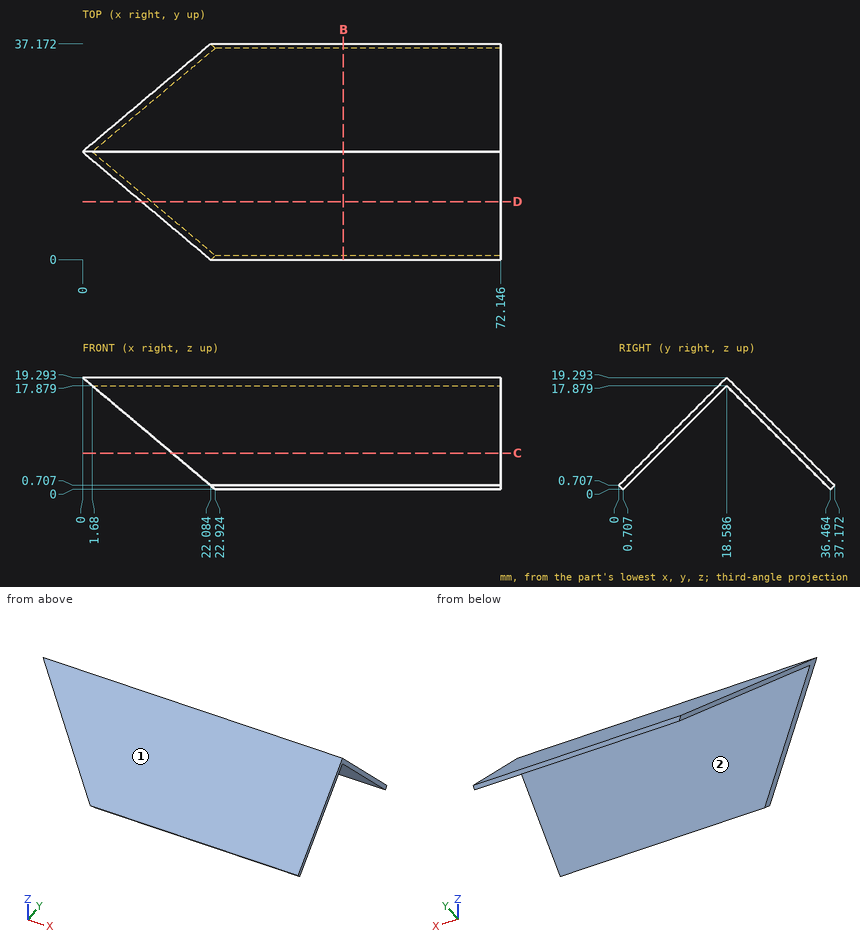
Check sheet for the drawn part. Datum: minimum x, y, z corner. Units: mm. Round coordinates to 2 decimals unless told otherwise and drop trailing zeros. Loops run counter-clockwise (first coordinate to the right, second up) from the corner with the lowest first, then second, coordinate; pieces in that order, holes last. Notation, with made-up numbers: (-8, 14.25) - (-3, 14.25) arc R22 cw to (-3, 46.25) - close; hole circle Ø4 at (19, -36.5). An arc over 180 degrees is marked (long way). Write item = value, one per line. Start each with the question number.
1. Mould release check, pull along Y, two halves, no side actions. Record for the marked faces 1 and 2: released by +Y, released by -Y, zero draft, split by the parting line, or undercut.
2. Section check C-C on z = 6.25. Enter the section's corners in (x, y) (1 decimal), then the cut area to 3 significant figures.
3. Thickness scan on line 1 (Y direction, x = 43, z = 16.5) (1 decimal); line 2 (Y direction, x = 58.5, z = 9.5) (1 decimal); line 3 (Z direction, x = 42, y = 2) (1 decimal). Record the ranges inside material, lowest first.
4. Depth check by flat-ended pin: pin 1 (6 mm diameter, centred on x = 56, z = 9, fed in from -Y); pin 2 (10 mm diameter, centred on x = 20.5, y = 24, fed in from -Z) (1 decimal); pin 3 (12 mm diameter, centred on x = 24, y = 4.5, fed in from +Z); pin 4 (1 mm diameter, centred on y = 14, z = 12, fed in from -X). Enter the tip coordinate at first touch or a pass-through.
5. Section check B-B on x = 45. Enter the section's corners in (y, z) (1 decimal).
6. Section check D-D on y = 10. Enter the section's corners in (x, z) (1 decimal).
Working result:
q1.face_1 = released by -Y
q1.face_2 = undercut
q2.outline = (15.5, 5.5) - (72.1, 5.5) - (72.1, 7) - (15.5, 7) - close; (15.5, 30.2) - (72.1, 30.2) - (72.1, 31.6) - (15.5, 31.6) - close
q2.area = 160 mm^2
q3.line_1 = 15.8 to 17.2, 20 to 21.4
q3.line_2 = 8.8 to 10.2, 27 to 28.4
q3.line_3 = 1.3 to 2.7
q4.pin_1 = 5.29
q4.pin_2 = 7.5
q4.pin_3 = 11.21
q4.pin_4 = through
q5.outline = (0, 0.7) - (0.7, 0) - (18.6, 17.9) - (36.5, 0) - (37.2, 0.7) - (18.6, 19.3) - close
q6.outline = (10.2, 10.7) - (11.9, 9.3) - (72.1, 9.3) - (72.1, 10.7) - close
